Model file for the job. Use its own axes, mm. A direction names the side the tool comes from. Give positions to 0.01 mm unless a question says otherwise; leave off trailing zeros. Loops run counter-clockwise (first coordinate to the right, second up) from the corner with the lowest first, then second, coordinate; pieces in that order, holes last. Notation, with made-up numbers: M 55,-17.5 L 62,-17.5 A31 cw 62,15.5 Z; hole C -1.5,86 d5. An arc over 180 degrees is marked long. Use CSV: the item, a comma, the result in double quotes. Start each with the question number.
(1) Slice it at D-D on z = 2.5. List the corners of the cut face in (x, y).
(2) Slice it at B-B on x = 22. List the corners of the cut face in (y, z).
(3) Slice it at A-A on z = 14.5. List the corners of the cut face in (x, y).
(4) Tool access for faces 1 (the face through (74, 0, 8)), 2 (the face through (-74, 0, 8)), 3 (the face through (0, 20, 9)), 4 (the face through (-1, -19, 4)), 5 (the face through (71, -11, 17)): list every direction of +Z, -Z, +X, -X, +Y, -Y with a clear straight run to the whole face (end or side of a thin tool).
(5) Wall check: line 1 along X through (y, z) = (-8.5, 12.75); line 2 along Y through (x, z) = (-22, 1.5); line 3 along X through (y, z) = (-0.5, 24.25). Give the ranges that are in metal, low to high. Write a range as from..to.
(6) Flat gauge pins, fed straight in: P1, Ø1.6, axis at x = -75.5, y = -1.5, coming from the -Z side; P2, Ø5, axis at x = 18.5, y = -17.5, coming from the +Z side; P3, Ø3, axis at x = -3, y = 16.5, coming from the +Z side; P4, Ø7, axis at x = 70.5, z = 20, coming from the +Y side. Where does each tip first touch, or does it go through?
(7) Slice it at C-C on y = -0.5. List the corners of the cut face in (x, z).
(8) Two-plate mould, pull along Y, no slides. Class faces 6 (the face through (-1, 19, 4)), 7 (the face through (72, 0, 25)), 8 (the face through (-71, -11, 17)): pulls with the +Y half, pulls with the -Y half, needs draft (parallel to the pull), parting line crosses it, or undercut.
```python
from build123d import *

# Parameters (mm, degrees)
F0_W     = 148
F0_H     = 43
F0_W_2   = 135
F0_H_2   = 38
F1_DEPTH = 9
F2_W     = 6.5
F2_H     = 22
F3_DEPTH = 16
F4_W     = 22
F4_H     = 3.5
F5_DEPTH = 2
F6_W     = 22
F6_H     = 3.5
F7_DEPTH = 2


with BuildPart() as f1:
    # F0 (on Top) → F1 (new body)
    with BuildSketch(Plane.XY):
        Rectangle(F0_W, F0_H)
        Rectangle(F0_W_2, F0_H_2, mode=Mode.SUBTRACT)
    extrude(amount=F1_DEPTH)

    # F2 (on face) → F3 (join)
    with BuildSketch(Plane.XY.offset(9)):
        with Locations((-70.75, 0)):
            Rectangle(F2_W, F2_H)
        with Locations((70.75, 0)):
            Rectangle(F2_W, F2_H)
    extrude(amount=F3_DEPTH)

    # F4 (on face) → F5 (join)
    with BuildSketch(Plane(origin=(-74, 0, 0), x_dir=(0, -1, 0), z_dir=(-1, 0, 0))):
        with Locations((0, 23.25)):
            Rectangle(F4_W, F4_H)
    extrude(amount=F5_DEPTH)

    # F6 (on face) → F7 (join)
    with BuildSketch(Plane.YZ.offset(74)):
        with Locations((0, 23.25)):
            Rectangle(F6_W, F6_H)
    extrude(amount=F7_DEPTH)


with BuildPart() as f8_1:
    # F8: copy of F1
    add(f1.part)


solid = f8_1.part
```
Reply:
1,outline,"M -74,-21.5 L 74,-21.5 L 74,21.5 L -74,21.5 Z; hole M -67.5,-19 L 67.5,-19 L 67.5,19 L -67.5,19 Z"
2,outline,"M -21.5,0 L -19,0 L -19,9 L -21.5,9 Z; M 19,0 L 21.5,0 L 21.5,9 L 19,9 Z"
3,outline,"M -74,-11 L -67.5,-11 L -67.5,11 L -74,11 Z; M 67.5,-11 L 74,-11 L 74,11 L 67.5,11 Z"
4,face 1,"-Z, +X, +Y, -Y"
4,face 2,"-Z, -X, +Y, -Y"
4,face 3,"+Z, +X, -X, +Y"
4,face 4,"+Z, -Z"
4,face 5,"+Z, +X, -X, -Y"
5,line 1,"x = -74..-67.5, 67.5..74"
5,line 2,"y = -21.5..-19, 19..21.5"
5,line 3,"x = -76..-67.5, 67.5..76"
6,P1,"stops at z = 21.5"
6,P2,"stops at z = 9"
6,P3,"passes through"
6,P4,"stops at y = 11"
7,outline,"M -76,21.5 L -74,21.5 L -74,0 L -67.5,0 L -67.5,25 L -76,25 Z; M 67.5,0 L 74,0 L 74,21.5 L 76,21.5 L 76,25 L 67.5,25 Z"
8,face 6,"undercut"
8,face 7,"needs draft"
8,face 8,"pulls with the -Y half"
